Part model, mm, in its own coordinate system. A direction names the side the tool comes from. Give positions to 0.01 mm unless a question says otherwise; leave off trailing zeros. Answer as a JSON object with one key per item and string values.
from build123d import *
from build123d import SkipClean  # not in build123d's __all__

# Parameters (mm, degrees)
F0_W      = 12
F0_H      = 12
F1_DEPTH  = 6
F2_R      = 4.7625
F3_DEPTH  = 1
F4_W      = 5
F4_H      = 5
F5_DEPTH  = 2
F6_SIZE   = 5
F7_SIZE   = 1.99999
F8_R      = 1
F10_DEPTH = 1
F12_DEPTH = 1
F13_R     = 3.25
F14_DEPTH = 7


# Not quite as in the source:
# - a fillet or chamfer is up to 0.001 mm smaller than in the source, because OpenCascade refuses the exact size


with BuildPart() as f1:
    # F0 (on Top) → F1 (new body)
    with BuildSketch(Plane.XY):
        with Locations((-6, 6)):
            Rectangle(F0_W, F0_H)
    extrude(amount=F1_DEPTH)

    # F2 (on face) → F3 (cut)
    with BuildSketch(Plane(origin=(0, 0, 0), x_dir=(1, 0, 0), z_dir=(0, 0, -1))):
        Circle(F2_R)
    extrude(amount=-F3_DEPTH, mode=Mode.SUBTRACT)

    # F4 (on face) → F5 (join)
    with BuildSketch(Plane.XY.offset(6)):
        with Locations((-2.5, 2.5)):
            Rectangle(F4_W, F4_H)
    extrude(amount=F5_DEPTH)

    # F6
    f6_edges = [f1.edges().sort_by_distance(p)[0] for p in [
        (-12, 6, 6),
        (-6, 12, 6),
    ]]
    chamfer(f6_edges, length=F6_SIZE)

    # F7 (size 2 in the source; OpenCascade refuses exactly that, so slightly less here)
    f7_edges = [f1.edges().sort_by_distance(p)[0] for p in [
        (-5, 5, 7),
        (-5, 2.5, 8),
        (-2.5, 5, 8),
    ]]
    chamfer(f7_edges, length=F7_SIZE)

    # F8
    f8_edges = [f1.edges().sort_by_distance(p)[0] for p in [
        (-7, 3.5, 6),
        (-3.5, 7, 6),
        (-9.5, 9.5, 3.5),
    ]]
    fillet(f8_edges, radius=F8_R)

    # F9 (on face) → F10 (cut)
    with BuildSketch(Plane(origin=(0, 6.5, 6.5), x_dir=(-1, 0, 0), z_dir=(0, 0.7071067812, 0.7071067812))):
        Polygon((0, -6.7781745931), (9.3610415662, -6.7781745931), (6.0681483474, -2.1213203436), (0, -2.1213203436), align=None)
    extrude(amount=-F10_DEPTH, mode=Mode.SUBTRACT)

    # F11 (on face) → F12 (cut)
    with BuildSketch(Plane(origin=(-6.5, 0, 6.5), x_dir=(0, -1, 0), z_dir=(-0.7071067812, 0, 0.7071067812))):
        Polygon((0, -6.7781745931), (0, -2.1213203436), (-6.0681483474, -2.1213203436), (-9.3610415662, -6.7781745931), align=None)
    extrude(amount=-F12_DEPTH, mode=Mode.SUBTRACT)

    # F13 (on face) → F14 (cut, through all)
    with BuildSketch(Plane.XY.offset(8)):
        Circle(F13_R)
    extrude(amount=-F14_DEPTH, mode=Mode.SUBTRACT)

    # F15: F1 across plane


with BuildPart() as f1_1:
    add(f1.part, clean=False)
    add(f1.part.mirror(Plane.XZ), clean=False)

    # F16: F1 across plane


with BuildPart() as f1_2:
    add(f1_1.part, clean=False)
    with SkipClean():  # cleaning this boolean's faces spoils the solid; the shape is the same uncleaned
        add(f1_1.part.mirror(Plane.YZ), clean=False)


solid = f1_2.part
1. Which spindle directions (+Z, -Z, +X, -X, +Y, -Y) get a long thin tool onto all of the face, cutting with end or side? Do faces 5 (the flat face through (6, 0, 6)), 6 (the cylindrical face through (9.457, -9.467, 3.349)). Say none if no direction does.
Worked answers:
{"face 5": "+Z", "face 6": "+Z, +X, -Y"}
2. Pin check, flat tips, straight feed: P1, Ø1, axis at x = 7.5, z = 3, coming from the -Y side; P2, Ø8, axis at x = -4, y = 7.5, coming from the +Z side; P3, Ø4, axis at x = -2.5, y = 1, coming from the -Z side. Stop position of each tip, or through.
Worked answers:
{"P1": "stops at y = -9.93", "P2": "stops at z = 7.37", "P3": "stops at z = 1"}
3. Two-plate mould, pull along Z, no slides. Class faces 1 (the flat face through (0.9, -11.4, 1.6)), 2 (the flat face through (-0.131, -8.916, 2.669)), 3 (the flat face through (12, 0.2, 0.5)), 4 (the flat face through (-7.74, -9.32, 2.98)): +Z half, -Z half, draft (parallel to the pull), parting line (faces both ways), or undercut.
Worked answers:
{"face 1": "+Z half", "face 2": "undercut", "face 3": "draft", "face 4": "undercut"}
4. Probe line 1 along Y through (x, z) = (-1.75, 7); line 2 along Z through (x, y) = (-7.5, -1); line 3 along X through (y, z) = (6.75, 1.25). List the from-to ranges inside material, lowest first.
Worked answers:
{"line 1": "y = -4 to -2.74, 2.74 to 4", "line 2": "z = 0 to 4.09, 4.5 to 5.5", "line 3": "x = -11.75 to -10.84, -10.34 to 10.34, 10.84 to 11.75"}
